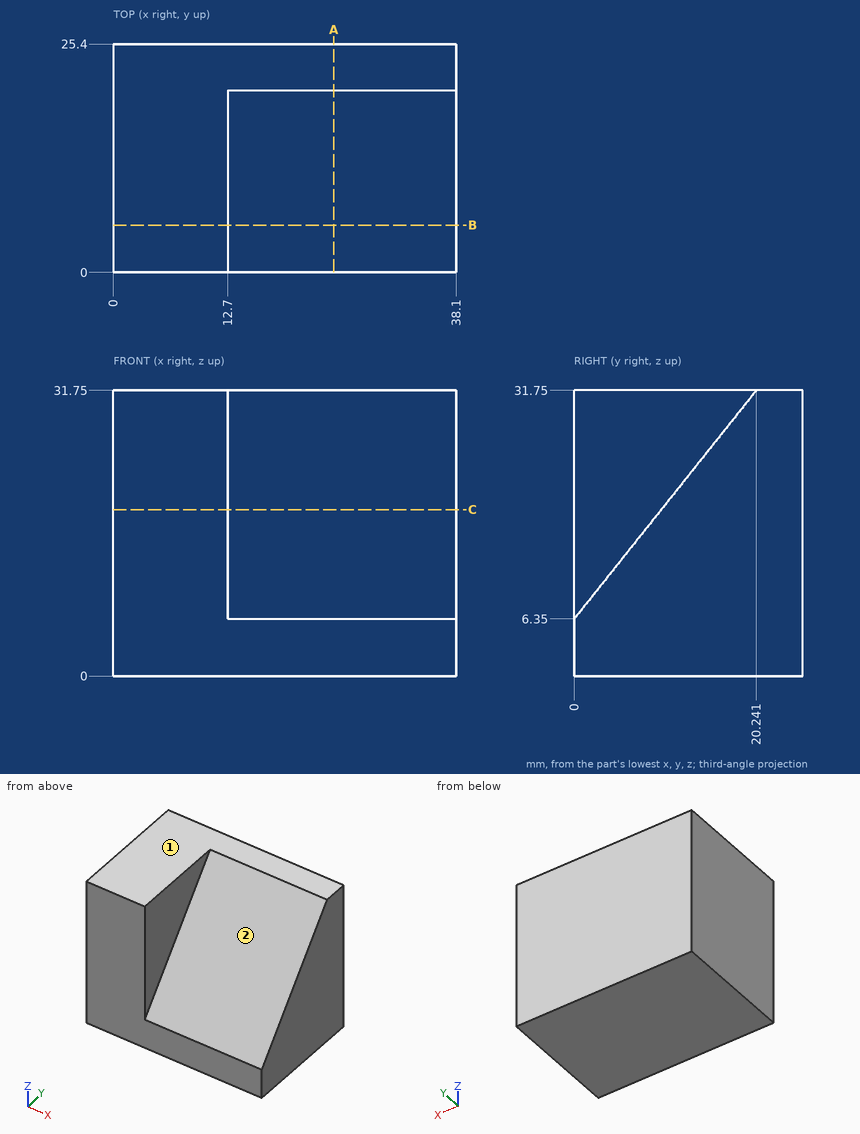
Verification items for this drawing (mm, ordinates from the low corner). A direction names the side the tool comes from. Round coordinates to 2 decimals unless told otherwise and drop trailing zeros. Order: outer loops, then holes, each group sorted by start corner. A loop starts at its lowest first (then second) coordinate and runs counter-clockwise, first axis right, second up. Notation, with made-up numbers: M 19.25,51 L 29.25,51 A5 ccw 29.25,58 Z; hole C -28,10.5 d4. An arc over 180 degrees is marked long. Answer in a Markdown table with one row per item. Add a question column.
Item 1: Depth check by flat-ended pin: pin 1 Ø6 at (x, z) = (26, 12) entering from -Y; pin 2 Ø10 at (y, z) = (5.5, 24.5) entering from +X; pin 3 Ø1.5 at (x, y) = (24, 18.5) entering from +Z. Enter the tip coordinate at first touch or a pass-through.
Item 2: Sectioned sample at B-B, the plane y = 5.25. Enter the section's corners in (x, z), plus the area to 3 significant figures.
Item 3: Sectioned sample at C-C, the plane z = 18.5. Enter the section's corners in (x, y).
Item 4: Material ranges on L1, parallel to X at y = 14, z = 24.5; L2, parallel to Z at x = 35.5, y = 6.5; L3, parallel to Y at x = 17, z = 13, recorded low to high. Write a range as [from, to].
Item 5: Sectioned sample at A-A, the plane x = 24.5. Enter the section's corners in (y, z), plus the area to 3 significant figures.
Item 6: Set-up check for the marked faces 1 and 2: record each of +Z, -Z, +X, -X, +Y, -Y from which the full face is reachable in a straight line by a thin tool's end or side.
Filled in:
| question | item | result |
|---|---|---|
| 1 | pin 1 | stops at y = 2.11 |
| 1 | pin 2 | stops at x = 12.7 |
| 1 | pin 3 | stops at z = 30.51 |
| 2 | outline | M 0,0 L 38.1,0 L 38.1,12.94 L 12.7,12.94 L 12.7,31.75 L 0,31.75 Z |
| 2 | area | 732 mm² |
| 3 | outline | M 0,0 L 12.7,0 L 12.7,9.68 L 38.1,9.68 L 38.1,25.4 L 0,25.4 Z |
| 4 | L1 | x = [0, 12.7] |
| 4 | L2 | z = [0, 14.51] |
| 4 | L3 | y = [5.3, 25.4] |
| 5 | outline | M 0,0 L 25.4,0 L 25.4,31.75 L 20.24,31.75 L 0,6.35 Z |
| 5 | area | 549 mm² |
| 6 | face 1 | +Z, +X, -X, +Y, -Y |
| 6 | face 2 | +Z, +X, -Y |
